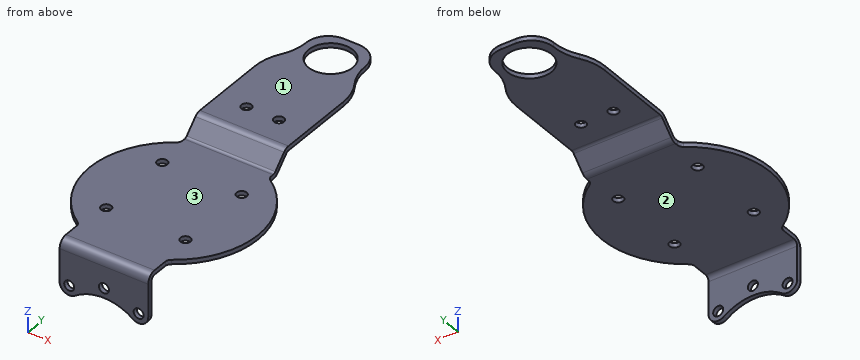
```python
from build123d import *

# Parameters (mm, degrees)
EXTRUDE_1_DEPTH             = 30
EXTRUDE_2_DEPTH             = 14.177345132
SKETCH_3_W                  = 30
SKETCH_3_H                  = 14.177345132
EXTRUDE_3_DEPTH             = 7.766758368
EXTRUDE_4_DEPTH             = 1.5
CUT_EXTRUDE_START           = -0.577345132
CUT_EXTRUDE_1_DEPTH         = 0.577345132
CUT_EXTRUDE_START_2         = -12.1
CUT_EXTRUDE_2_DEPTH         = 12.1
SKETCH_7_W                  = 30
SKETCH_7_H                  = 7
EXTRUDE_5_DEPTH             = 52.621320344
CUT_EXTRUDE_3_DEPTH         = 97.803565652
CUT_EXTRUDE_4_DEPTH         = 93.536010044
CUT_EXTRUDE_5_DEPTH         = 93.536010044
HOLE_WIZARD_3_4_3_4_1_D     = 3.4
HOLE_WIZARD_3_4_3_4_2_D     = 3.4
HOLE_WIZARD_15_0_15_1_D     = 15
HOLE_WIZARD_3_4_3_4_3_D     = 3.4
HOLE_WIZARD_3_4_3_4_3_DEPTH = 17.427345132
FILLET_1_R                  = 1.5
FILLET_2_R                  = 2
FILLET_3_R                  = 3
FILLET_4_R                  = 7.5


with BuildPart() as part:
    # 草图1 → 凸台-拉伸1 (new body)
    with BuildSketch(Plane(origin=(15, 0, 0), x_dir=(0, 0, -1), z_dir=(1, 0, 0))):
        Polygon((-7, 32.378679656), (-1.5, 26.878679656), (-1.5, 32.378679656), align=None)
    extrude(amount=-EXTRUDE_1_DEPTH)

    # 草图2 → 凸台-拉伸2 (add)
    with BuildSketch(Plane(origin=(0, 0, 1.5), x_dir=(-1, 0, 0), z_dir=(0, 0, -1))):
        with BuildLine():
            Line((-15, 24.233241632), (-15, 32.378679656))
            Line((-15, 32.378679656), (15, 32.378679656))
            Line((15, 32.378679656), (15, 24.233241632))
            ThreePointArc((15, 24.233241632), (28.5, 0), (15, -24.233241632))
            Line((15, -24.233241632), (-15, -24.233241632))
            ThreePointArc((-15, -24.233241632), (-28.5, 0), (-15, 24.233241632))
        make_face()
    extrude(amount=EXTRUDE_2_DEPTH)

    # 草图3 → 凸台-拉伸3 (add)
    with BuildSketch(Plane.XZ.offset(24.233241632)):
        with Locations((0, -5.588672566)):
            Rectangle(SKETCH_3_W, SKETCH_3_H)
    extrude(amount=EXTRUDE_3_DEPTH)

    # 草图4 → 凸台-拉伸4 (add)
    with BuildSketch(Plane.XZ.offset(32)):
        with BuildLine():
            Line((15, 1.5), (15, -12.677345132))
            ThreePointArc((15, -12.677345132), (13.223342916, -15.57419871), (9.835839599, -15.303842792))
            ThreePointArc((9.835839599, -15.303842792), (0, -12.1), (-9.835839599, -15.303842792))
            ThreePointArc((-9.835839599, -15.303842792), (-13.223342916, -15.57419871), (-15, -12.677345132))
            Line((-15, -12.677345132), (-15, 1.5))
            Line((-15, 1.5), (15, 1.5))
        make_face()
    extrude(amount=EXTRUDE_4_DEPTH)

    # 草图5 → 切除-拉伸1 (cut)
    with BuildSketch(Plane(origin=(0, 0, -12.677345132), x_dir=(-1, 0, 0), z_dir=(0, 0, -1)).offset(CUT_EXTRUDE_START)):
        with BuildLine():
            Line((15, 24.233241632), (15, 32.378679656))
            Line((15, 32.378679656), (-15, 32.378679656))
            Line((-15, 32.378679656), (-15, 24.233241632))
            ThreePointArc((-15, 24.233241632), (-28.5, 0), (-15, -24.233241632))
            Line((-15, -24.233241632), (-15, -32))
            Line((-15, -32), (0, -32))
            Line((0, -32), (15, -32))
            Line((15, -32), (15, -24.233241632))
            ThreePointArc((15, -24.233241632), (28.5, 0), (15, 24.233241632))
        make_face()
    extrude(amount=CUT_EXTRUDE_1_DEPTH, mode=Mode.SUBTRACT)

    # 草图6 → 切除-拉伸2 (cut)
    with BuildSketch(Plane(origin=(0, 0, -12.1), x_dir=(-1, 0, 0), z_dir=(0, 0, -1)).offset(CUT_EXTRUDE_START_2)):
        with BuildLine():
            Line((15, 24.233241632), (15, 32.378679656))
            Line((15, 32.378679656), (-15, 32.378679656))
            Line((-15, 32.378679656), (-15, 24.233241632))
            ThreePointArc((-15, 24.233241632), (-28.5, 0), (-15, -24.233241632))
            Line((-15, -24.233241632), (-15, -32))
            Line((-15, -32), (15, -32))
            Line((15, -32), (15, -24.233241632))
            ThreePointArc((15, -24.233241632), (28.5, 0), (15, 24.233241632))
        make_face()
    extrude(amount=CUT_EXTRUDE_2_DEPTH, mode=Mode.SUBTRACT)

    # 草图7 → 凸台-拉伸5 (add)
    with BuildSketch(Plane(origin=(0, 32.378679656, 0), x_dir=(-1, 0, 0), z_dir=(0, 1, 0))):
        with Locations((0, 3.5)):
            Rectangle(SKETCH_7_W, SKETCH_7_H)
    extrude(amount=EXTRUDE_5_DEPTH)

    # 草图8 → 切除-拉伸3 (cut, through all)
    with BuildSketch(Plane.ZY.offset(15)):
        Polygon((0, 27.5), (5.5, 33), (5.5, 85), (0, 85), align=None)
    extrude(amount=-CUT_EXTRUDE_3_DEPTH, mode=Mode.SUBTRACT)

    # 草图9 → 切除-拉伸4 (cut, through all)
    with BuildSketch(Plane.XY.offset(7)):
        with BuildLine():
            Line((-11.795428312, 85), (-15, 85))
            Line((-15, 85), (-15, 60))
            ThreePointArc((-15, 60), (-14.362740383, 64.550068681), (-12.5, 68.75))
            ThreePointArc((-12.5, 68.75), (-10.015546325, 76.782552918), (-11.795428312, 85))
        make_face()
    extrude(amount=-CUT_EXTRUDE_4_DEPTH, mode=Mode.SUBTRACT)

    # 草图10 → 切除-拉伸5 (cut, through all)
    with BuildSketch(Plane.XY.offset(7)):
        with BuildLine():
            Line((15, 60), (15, 85))
            Line((15, 85), (11.795428312, 85))
            ThreePointArc((11.795428312, 85), (10.015546325, 76.782552918), (12.5, 68.75))
            ThreePointArc((12.5, 68.75), (14.362740383, 64.550068681), (15, 60))
        make_face()
    extrude(amount=-CUT_EXTRUDE_5_DEPTH, mode=Mode.SUBTRACT)

    # Ø3.4 (3.4) 直径孔1 (through all)
    with Locations(Plane(origin=(0, 0, 5.5), x_dir=(-1, 0, 0), z_dir=(0, 0, -1))):
        with Locations((5.5, 42.5), (-5.5, 42.5)):
            Hole(HOLE_WIZARD_3_4_3_4_1_D / 2)

    # Ø3.4 (3.4) 直径孔2 (through all)
    with Locations(Plane(origin=(0, -32, 0), x_dir=(1, 0, 0), z_dir=(0, 1, 0))):
        with Locations((-11.75, 12.677345132), (0, 8.85), (11.75, 12.677345132)):
            Hole(HOLE_WIZARD_3_4_3_4_2_D / 2)

    # Ø15.0 (15) 直径孔1 (through all)
    with Locations(Plane(origin=(0, 0, 5.5), x_dir=(-1, 0, 0), z_dir=(0, 0, -1))):
        with Locations((0, 75)):
            Hole(HOLE_WIZARD_15_0_15_1_D / 2)

    # Ø3.4 (3.4) 直径孔3
    with Locations(Plane.XY.offset(1.5)):
        with Locations((-13.435028843, -13.435028843), (-13.435028843, 13.435028843), (13.435028843, -13.435028843), (13.435028843, 13.435028843)):
            Hole(HOLE_WIZARD_3_4_3_4_3_D / 2, depth=HOLE_WIZARD_3_4_3_4_3_DEPTH)

    # 圆角1
    fillet_1_edges = [part.edges().sort_by_distance(p)[0] for p in [
        (0, -32, 0),
        (0, 33, 5.5),
        (0, 26.878679656, 1.5),
    ]]
    fillet(fillet_1_edges, radius=FILLET_1_R)

    # 圆角2
    fillet_2_edges = [part.edges().sort_by_distance(p)[0] for p in [
        (-15, -24.233241632, 0.75),
        (15, -24.233241632, 0.75),
        (-15, 24.233241632, 0.75),
        (15, 24.233241632, 0.75),
    ]]
    fillet(fillet_2_edges, radius=FILLET_2_R)

    # 圆角3
    fillet_3_edges = [part.edges().sort_by_distance(p)[0] for p in [
        (0, 27.5, 0),
        (0, -33.5, 1.5),
        (0, 32.378679656, 7),
    ]]
    fillet(fillet_3_edges, radius=FILLET_3_R)

    # 圆角4
    fillet_4_edges = [part.edges().sort_by_distance(p)[0] for p in [
        (-11.795428312, 85, 6.25),
        (11.795428312, 85, 6.25),
    ]]
    fillet(fillet_4_edges, radius=FILLET_4_R)


solid = part.part
```
The model under review builds one solid part; all positions refer to its coordinate system, in mm. Face numbers are marked on the shaded views. A direction names the side the tool comes from. Coordinates: 2 decimals unless noted, no trailing zeros. Write each loop counter-clockwise with the first axis right and the second up, starting at its lowest first coordinate (ties: lowest second). Pieces come first, ordered by that corner, then holes. Notation, with made-up numbers: (-10, 36) - (30, 36) arc R24 ccw to (30, 61) - close; hole circle Ø5 at (9, -10.75). An arc over 180 degrees is marked (long way). Answer in a Markdown table with one row per item. Add a question column.
Q1. Clearance check with flat-ended pins moving along their axes: pin 1 (12 mm diameter, centred on x = -12.5, y = 7.5, fed in from -Z); pin 2 (2 mm diameter, centred on x = 7.5, z = -2.5, fed in from +Y); pin 3 (7.5 mm diameter, centred on y = 48, z = 4, fed in from +X). State where each tip first meets the part, or that it passes through.
Q2. For the marked faces 1, 2 and 3, list the 3-axis set-ups (+Z, -Z, +X, -X, +Y, -Y) from which the entire face can be reached by the end or side of a thin tool; tool diameter is ignored.
Q3. Consider section D-D on y = 9. Give the boundary of the cut face in (x, z), then the cut area to 3 significant figures.
Q4. To check wall thickness, follow line 1 along X through (y, z) = (-32.7, -8.85); line 2 along Z through (x, y) = (2, 34); line 3 along Y through (x, z) = (-5.5, 5.85). State the ranges of each line that lie inside material, in increasing order. Write a range as from..to.
Q5. Consider section A-A on z = -8.85. Give the boundary of the cut face in (x, y), then the cut area to 3 significant figures.
Q6. Consider section C-C on y = 70. Give the boundary of the cut face in (x, z).
Q7. Consider section B-B on x = 0. Give the boundary of the cut face in (y, z), then the cut area to 3 significant figures.
Answers below:
| question | item | result |
|---|---|---|
| 1 | pin 1 | z = 0 |
| 1 | pin 2 | y = -32 |
| 1 | pin 3 | x = 15 |
| 2 | face 1 | +Z, +X, -X, +Y, -Y |
| 2 | face 2 | -Z, +X, -X, +Y |
| 2 | face 3 | +Z, +X, -X, -Y |
| 3 | outline | (-27.04, 0) - (27.04, 0) - (27.04, 1.5) - (-27.04, 1.5) - close |
| 3 | area | 81.1 mm² |
| 4 | line 1 | -15..-1.7, 1.7..15 |
| 4 | line 2 | 5.5..7 |
| 4 | line 3 | 31.23..40.8, 44.2..69.9, 80.1..84.37 |
| 5 | outline | (-15, -33.5) - (-1.7, -33.5) - (-1.7, -32) - (-15, -32) - close; (1.7, -33.5) - (15, -33.5) - (15, -32) - (1.7, -32) - close |
| 5 | area | 39.9 mm² |
| 6 | outline | (-11.8, 5.5) - (-5.59, 5.5) - (-5.59, 7) - (-11.8, 7) - close; (5.59, 5.5) - (11.8, 5.5) - (11.8, 7) - (5.59, 7) - close |
| 7 | outline | (-33.5, -12.1) - (-32, -12.1) - (-32, -10.55) - (-33.5, -10.55) - close; (-33.5, -7.15) - (-32, -7.15) - (-32, -1.5) arc R1.5 cw to (-30.5, 0) - (26.26, 0) arc R3 ccw to (28.38, 0.88) - (32.56, 5.06) arc R1.5 cw to (33.62, 5.5) - (67.5, 5.5) - (67.5, 7) - (33.62, 7) arc R3 ccw to (31.5, 6.12) - (27.32, 1.94) arc R1.5 cw to (26.26, 1.5) - (-30.5, 1.5) arc R3 ccw to (-33.5, -1.5) - close; (82.5, 5.5) - (85, 5.5) - (85, 7) - (82.5, 7) - close |
| 7 | area | 170 mm² |
